Verification items for the finished model (mm, model axes). A direction names the side the tool comes from. Coordinates: 2 decimals unless noted, no trailing zeros. Order: outer loops, then holes, each group sorted by start corner. A loop starts at its lowest first (then second) coordinate and runs counter-clockwise, first axis right, second up. Notation, with made-up numbers: M 68,22 L 114,22 A25 cw 114,47 Z; hole C 18,63 d1. An arc over 180 degrees is marked long. Return JSON: item names as keys, results as strings.
```python
from build123d import *

# Parameters (mm, degrees)
SKETCH1_R                = 101.6
BOSS_EXTRUDE1_DEPTH      = 27.813
BOSS_EXTRUDE2_DEPTH      = 55.626
BOSS_EXTRUDE2_DEPTH_BACK = 124.206
SKETCH2_R                = 9.525
FILLET1_R                = 20.32


with BuildPart() as part:
    # Sketch1 → Boss-Extrude1 (new, symmetric)
    with BuildSketch(Plane(origin=(0, 0, 0), x_dir=(1, 0, 0), z_dir=(0, 1, 0))):
        with Locations(Location((0, 0, 0), (0, 0, 270))):
            Circle(SKETCH1_R)
    extrude(amount=BOSS_EXTRUDE1_DEPTH, both=True)

    # Sketch2 → Boss-Extrude2 (add, two sides: drawn at the far end of the back side and taken through both)
    with BuildSketch(Plane(origin=(0, 27.813, 0), x_dir=(1, 0, 0), z_dir=(0, 1, 0)).offset(-BOSS_EXTRUDE2_DEPTH_BACK)):
        with Locations(Location((0, 0, 0), (0, 0, 270))):
            Circle(SKETCH2_R)
    extrude(amount=BOSS_EXTRUDE2_DEPTH + BOSS_EXTRUDE2_DEPTH_BACK)

    # Fillet1
    fillet1_edges = [part.edges().sort_by_distance(p)[0] for p in [
        (0, -27.813, -101.6),
        (0, 27.813, -101.6),
    ]]
    fillet(fillet1_edges, radius=FILLET1_R)


solid = part.part
```
Q1. Material ranges on line 1 along Y through (x, z) = (22.5, 6.5); line 2 along Y through (x, z) = (-73.5, 40.5); line 3 along Z through (x, y) = (-15.5, -13), recorded low to high.
Values:
{"line 1": "-27.81 to 27.81", "line 2": "-27.64 to 27.64", "line 3": "-99.64 to 99.64"}
Q2. Go/stop test with flat-tipped pins: pin 1 (3 mm diameter, centred on x = -4, y = -40.5, fed in from -Z); pin 2 (6 mm diameter, centred on x = -36, z = 76.5, fed in from -Y); pin 3 (1.5 mm diameter, centred on x = 0, y = 61.5, fed in from +Z) (3 decimals). Record where each tip stops, or that it passes through.
Values:
{"pin 1": "z = -9.19", "pin 2": "y = -27.81", "pin 3": "z = 9.525"}
Q3. Cross-section at D-D, the plane y = -15. Record the boundary of the cut face in (x, z).
Values:
{"outline": "C 0,0 d200.32"}
Q4. Cross-section at C-C, the plane y = 44. Record the boundary of the cut face in (x, z) (3 decimals).
Values:
{"outline": "C 0,0 d19.05"}
Q5. Tool access check on faces 1 (the face through (-5.796, -62.583, -7.559)), 2 (the face through (-5.796, 55.237, -7.559)), 3 (the face through (0, -96.393, 0)). Record the directions out of +Z, -Z, +X, -X, +Y, -Y that give a thin tool (end or side, any length) a straight path to the whole face; none if there is none.
Values:
{"face 1": "-Y", "face 2": "+Y", "face 3": "+Z, -Z, +X, -X, -Y"}
Q6. Cross-section at B-B, the plane x = 0. Record the boundary of the cut face in (y, z) (3 decimals).
Values:
{"outline": "M -96.393,-9.525 L -27.813,-9.525 L -27.813,-81.28 A20.32 ccw -7.493,-101.6 L 7.493,-101.6 A20.32 ccw 27.813,-81.28 L 27.813,-9.525 L 83.439,-9.525 L 83.439,9.525 L 27.813,9.525 L 27.813,81.28 A20.32 ccw 7.493,101.6 L -7.493,101.6 A20.32 ccw -27.813,81.28 L -27.813,9.525 L -96.393,9.525 Z"}
Q7. Cross-section at A-A, the plane z = 0. Record the boundary of the cut face in (x, y) (3 decimals), and give its area (3 significant figures).
Values:
{"outline": "M -101.6,-7.493 A20.32 ccw -81.28,-27.813 L -9.525,-27.813 L -9.525,-96.393 L 9.525,-96.393 L 9.525,-27.813 L 81.28,-27.813 A20.32 ccw 101.6,-7.493 L 101.6,7.493 A20.32 ccw 81.28,27.813 L 9.525,27.813 L 9.525,83.439 L -9.525,83.439 L -9.525,27.813 L -81.28,27.813 A20.32 ccw -101.6,7.493 Z", "area": "13,300 mm^2"}
